Job drawing, mm, ordinate dimensions from the low corner. One solid piece. A direction names the side the tool comes from. Give positions to 0.01 mm unless a question says otherwise; leave off trailing zeros. Order: outer loops, then holes, each group sorted by start corner. A loop starts at its lowest first (then second) coordinate and runs counter-clockwise, first axis right, second up. Notation, with made-up numbers: M 21.25,-8.75 L 65.25,-8.75 A20 ccw 65.25,30.25 Z; hole C 27.5,-7 d2. An arc over 180 degrees is marked long. One line per item, written item: value. Start each with the question number.
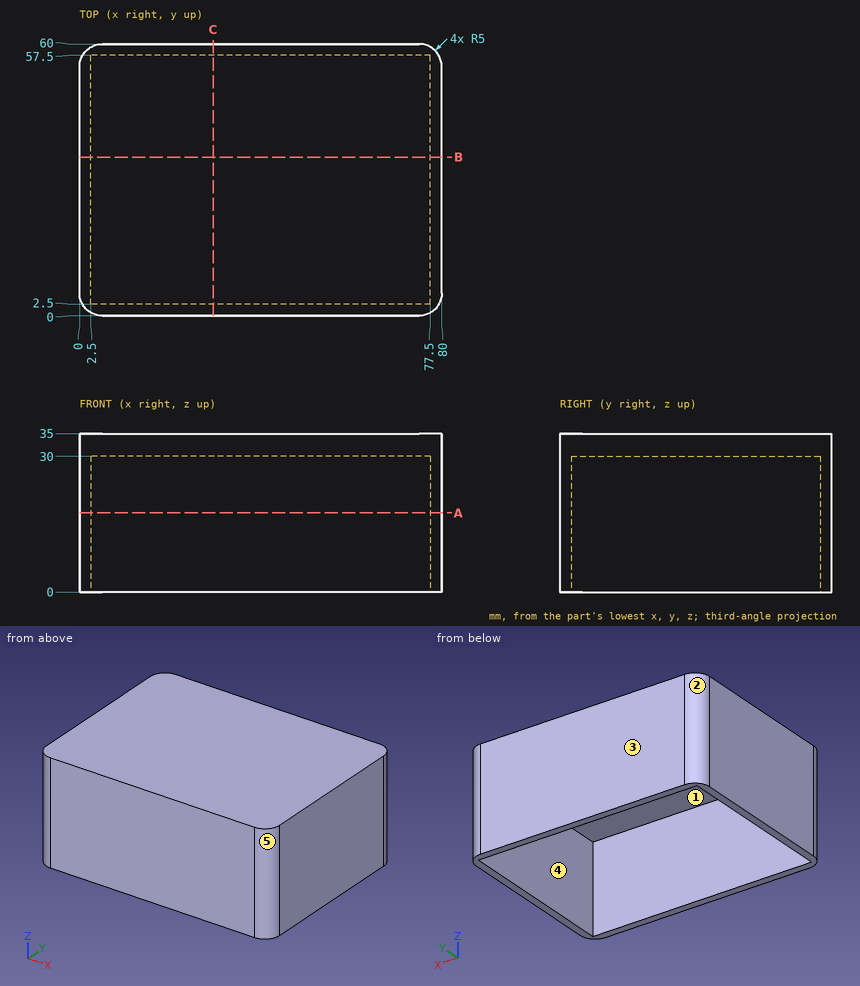
1) Slice it at C-C (x = 29.5). List the corners of the cut face in (y, z), plus the area to 3 significant figures.
2) Drop a flat-ended pin along its axis: P1, Ø1.5, axis at x = 55.5, y = 45, coming from the -Z side. Give the stop position or say it passes through.
3) Slice it at B-B (y = 35). List the corners of the cut face in (x, z).
4) Pull direction X, two halves, no side cores. Call the marked faces 1, 2 and 3: pulls with the +X half, pulls with the -X half, needs draft (parallel to the pull), parting line crosses it, or undercut.
5) Slice it at A-A (z = 17.5). List the corners of the cut face in (x, y).
6) Drill centre lines: line 1 (X direction, y = 53, z = 7); line 2 (Y direction, x = 6, z = 3); line 3 (Z direction, x = 60.5, y = 24). Where is each one in solid material? Low to high.
7) Tool access for the marked faces 4 and 5: list every direction of +Z, -Z, +X, -X, +Y, -Y with a clear straight run to the whole face (end or side of a thin tool).
Results list:
1. outline: M 0,0 L 2.5,0 L 2.5,30 L 57.5,30 L 57.5,0 L 60,0 L 60,35 L 0,35 Z
1. area: 450 mm²
2. P1: stops at z = 30
3. outline: M 0,0 L 2.5,0 L 2.5,30 L 77.5,30 L 77.5,0 L 80,0 L 80,35 L 0,35 Z
4. face 1: undercut
4. face 2: pulls with the -X half
4. face 3: needs draft
5. outline: M 0,5 A5 ccw 5,0 L 75,0 A5 ccw 80,5 L 80,55 A5 ccw 75,60 L 5,60 A5 ccw 0,55 Z; hole M 2.5,2.5 L 77.5,2.5 L 77.5,57.5 L 2.5,57.5 Z
6. line 1: x = 0 to 2.5, 77.5 to 80
6. line 2: y = 0 to 2.5, 57.5 to 60
6. line 3: z = 30 to 35
7. face 4: -Z
7. face 5: +Z, -Z, +X, -Y
